from build123d import *

# Parameters (mm, degrees)
F0_R            = 21.075
F0_R_2          = 11.075
F1_DEPTH        = 7
F4_DEPTH        = 12.5
F4_COPIES_COUNT = 12


# Not quite as in the source:
# - a pattern or mirror of a feature is missing from the dataset's text; its kind, count and spacing are read off the source's solid


with BuildPart() as f1:
    # F0 (on Top) → F1 (new body)
    with BuildSketch(Plane.XY):
        Circle(F0_R)
        Circle(F0_R_2, mode=Mode.SUBTRACT)
    extrude(amount=F1_DEPTH)

    # F3 (on offset) → F4 (cut)
    with BuildSketch(Plane.XZ.offset(25)):
        with BuildLine():
            Line((0, 1), (0, 6))
            ThreePointArc((0, 6), (-2.5, 3.5), (0, 1))
        make_face()
        with BuildLine():
            ThreePointArc((0, 1), (1.767766953, 1.732233047), (2.5, 3.5))
            ThreePointArc((2.5, 3.5), (1.767766953, 5.267766953), (0, 6))
            Line((0, 6), (0, 1))
        make_face()
    f4 = extrude(amount=-F4_DEPTH, mode=Mode.SUBTRACT)

    # F4_copies: F4 ×12 about axis
    f4_copies_axis = Axis((0, 0, 0), (0, 0, 1))
    for i in range(1, F4_COPIES_COUNT):
        add(f4.rotate(f4_copies_axis, i * 360 / F4_COPIES_COUNT), mode=Mode.SUBTRACT)


solid = f1.part
Geometry: final body of the model. Coordinates: model frame, mm. A direction names the side the tool comes from. Give positions to 0.01 mm unless a question says otherwise; leave off trailing zeros. Write each loop counter-clockwise with the first axis right and the second up, starting at its lowest first coordinate (ties: lowest second). Pieces come first, ordered by that corner, then holes.
(1) Ray query, line 1 (Y direction, x = 0, z = 2.25) (3 decimals); line 2 (X direction, y = 15.5, z = 3.75); line 3 (Y direction, x = -11.5, z = 2.75). Return the intervals inside material, ascending.
(2) Cut plane D-D, the plane y = 5. Give the number of separate pieces and of enclosed holes in the cut face, then the cut area to 3 significant figures.
(3) Cut plane B-B, the plane x = -1.5. Return loops of the section in (y, z), then the cut area to 3 significant figures.
(4) Access query for faces 5 (the flat face through (-12.5, 0, 4)), 6 (the flat face through (-6.28, -10.81, 3.54)), 7 (the cylindrical face through (-2.4, -10.81, 3.45)), 8 (the flat face through (0, -12.5, 4)), 9 (the flat face through (12.5, 0, 4)). Directions: +Z, -Z, +X, -X, +Y, -Y. A direction counts if a zero-diameter tool reaches every point of the face in a straight line with its end or side. Return the directions, or none.
(5) Cut plane A-A, the plane y = -3.5. Return loops of the section in (x, z), then the cut area to 3 significant figures.
(6) Cut plane C-C, the plane z = 6.5. Return loops of the section in (x, y) (3 decimals).
(7) Mould query, pull axis X, two halves, no side actions, for faces 1 (the flat face through (0, 12.5, 4)), 2 (the flat face through (9, -9, 0)), 3 (the cylindrical face through (-15.533, 14.243, 3.451)), 4 (the flat face through (-10.81, 6.28, 3.54)). Classes: released by +X, released by -X, zero draft, split by the parting line, or undercut.
(8) First-contact query: P1, Ø4, axis at x = 0.5, z = 2.5, coming from the +Y side (3 decimals); P2, Ø1.5, axis at y = 0, z = 3.5, coming from the +X side; P3, Ø1.5, axis at x = -1, z = 3.5, coming from the -Y side; P4, Ø13.5, axis at x = 0, y = 0, coming from the -Z side. Flat tips, straight axial feed; report the tip coordinate or a pass-through.
Values follow:
1. line 1: y = -12.5 to -11.075, 11.075 to 12.5
1. line 2: x = -14.28 to -11.82, -6.08 to -2.49, 2.49 to 6.08, 11.82 to 14.28
1. line 3: y = -15.15 to -9.39, -5.08 to 5.08, 9.39 to 15.15
2. separate pieces: 2
2. enclosed holes: 2
2. area: 136 mm2
3. outline: (-21.02, 0) - (-10.97, 0) - (-10.97, 7) - (-21.02, 7) - (-21.02, 5.5) - (-12.5, 5.5) - (-12.5, 1.5) - (-21.02, 1.5) - close; (10.97, 0) - (21.02, 0) - (21.02, 1.5) - (12.5, 1.5) - (12.5, 5.5) - (21.02, 5.5) - (21.02, 7) - (10.97, 7) - close
3. area: 72.5 mm2
4. face 5: -X
4. face 6: none
4. face 7: +Z, -Z
4. face 8: -Y
4. face 9: +X
5. outline: (-20.78, 0) - (-10.51, 0) - (-10.51, 7) - (-20.78, 7) - close; (10.51, 0) - (20.78, 0) - (20.78, 7) - (10.51, 7) - close
5. area: 144 mm2
6. outline: circle Ø42.15 at (0, 0); hole circle Ø22.15 at (0, 0)
7. face 1: undercut
7. face 2: zero draft
7. face 3: split by the parting line
7. face 4: undercut
8. P1: stops at y = 21.075
8. P2: stops at x = 12.5
8. P3: stops at y = -12.5
8. P4: passes through
